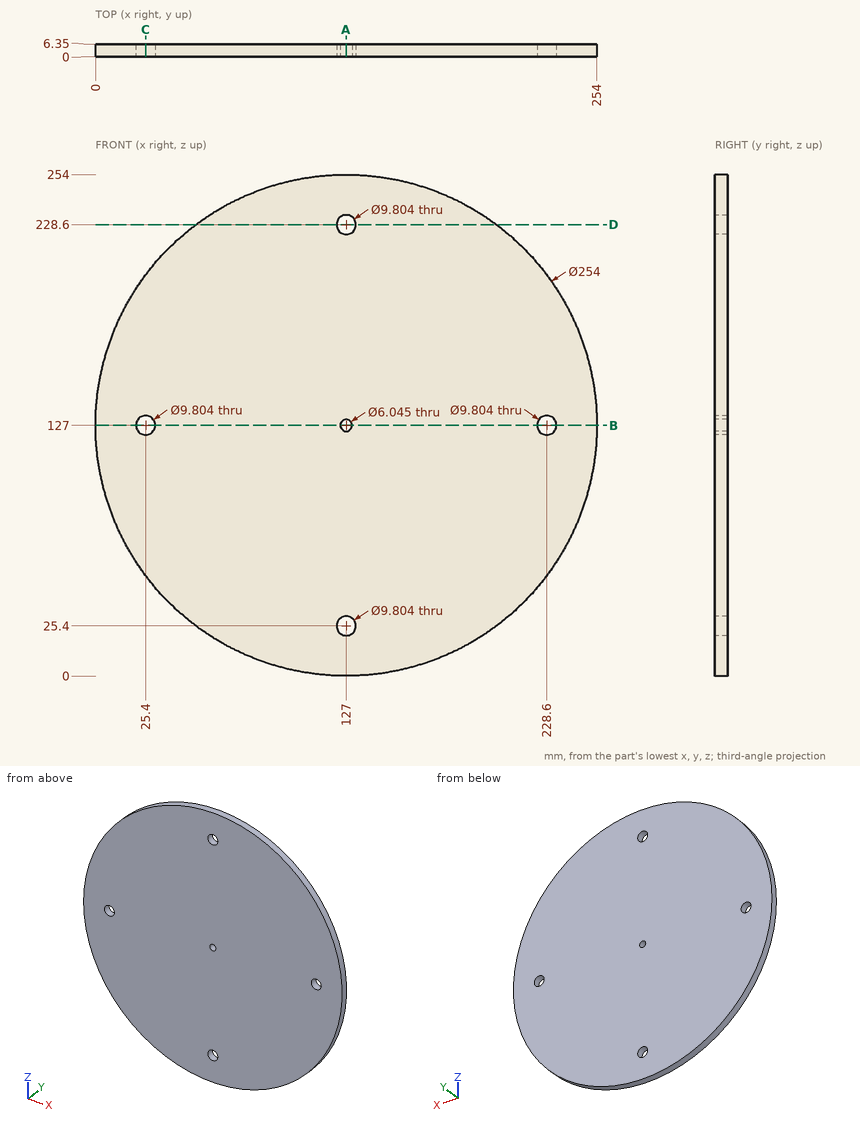
Verification items for this drawing (mm, ordinates from the low corner). Give positions to 0.01 mm unless a question says otherwise; leave off trailing zeros. Write each loop counter-clockwise with the first axis right and the second up, starting at its lowest first coordinate (ties: lowest second). Pieces come first, ordered by that corner, then holes. Notation, with made-up numbers: (-22, 17) - (18, 17) arc R33 cw to (18, 52) - close; hole circle Ø7 at (-9, 77). An arc over 180 degrees is marked (long way). Answer as CSV lines item,"result". Start each with the question number.
1. Sectioned sample at A-A (x = 127). Record the boundary of the cut face in (y, z).
2. Thickness scan on line 1 (Z direction, x = 127, y = 4); line 2 (X direction, y = 4.25, z = 125.5) (1 decimal); line 3 (Z direction, x = 228.6, y = 4.5) (1 decimal). Record the ranges inside material, lowest first.
3. Sectioned sample at D-D (z = 228.6). Record the boundary of the cut face in (x, y).
4. Sectioned sample at C-C (x = 25.4). Record the boundary of the cut face in (y, z).
5. Sectioned sample at B-B (z = 127). Record the boundary of the cut face in (x, y), then the cut area to 3 significant figures.
6. Depth check by flat-ended pin: pin 1 (3 mm diameter, centred on x = 158, y = 4, fed in from +Z); pin 2 (1 mm diameter, centred on x = 174.5, y = 5.5, fed in from -Z); pin 3 (2 mm diameter, centred on y = 4.5, z = 122, fed in from -X). Enter the tip coordinate at first touch or a pass-through.
Derived:
1,outline,"(0, 0) - (6.35, 0) - (6.35, 20.5) - (0, 20.5) - close; (0, 30.3) - (6.35, 30.3) - (6.35, 123.98) - (0, 123.98) - close; (0, 130.02) - (6.35, 130.02) - (6.35, 223.7) - (0, 223.7) - close; (0, 233.5) - (6.35, 233.5) - (6.35, 254) - (0, 254) - close"
2,line 1,"0 to 20.5, 30.3 to 123.98, 130.02 to 223.7, 233.5 to 254"
2,line 2,"0 to 20.7, 30.1 to 124.4, 129.6 to 223.9, 233.3 to 254"
2,line 3,"50.8 to 122.1, 131.9 to 203.2"
3,outline,"(50.8, 0) - (122.1, 0) - (122.1, 6.35) - (50.8, 6.35) - close; (131.9, 0) - (203.2, 0) - (203.2, 6.35) - (131.9, 6.35) - close"
4,outline,"(0, 50.8) - (6.35, 50.8) - (6.35, 122.1) - (0, 122.1) - close; (0, 131.9) - (6.35, 131.9) - (6.35, 203.2) - (0, 203.2) - close"
5,outline,"(0, 0) - (20.5, 0) - (20.5, 6.35) - (0, 6.35) - close; (30.3, 0) - (123.98, 0) - (123.98, 6.35) - (30.3, 6.35) - close; (130.02, 0) - (223.7, 0) - (223.7, 6.35) - (130.02, 6.35) - close; (233.5, 0) - (254, 0) - (254, 6.35) - (233.5, 6.35) - close"
5,area,"1,450 mm²"
6,pin 1,"z = 250.53"
6,pin 2,"z = 9.02"
6,pin 3,"x = 0.06"
